```python
from build123d import *

# Parameters (mm, degrees)
CYLINDER042_R     = 3.15
CYLINDER042_DEPTH = 10
ARRAY016_Y_COUNT  = 2
ARRAY016_Y_PITCH  = 51.7
CYLINDER036_R     = 2.2
CYLINDER036_DEPTH = 26
ARRAY010_X_COUNT  = 2
ARRAY010_X_PITCH  = 11.9
ARRAY010_Y_COUNT  = 3
ARRAY010_Y_PITCH  = 7.5
CYLINDER035_R     = 2.2
CYLINDER035_DEPTH = 26
ARRAY009_X_COUNT  = 2
ARRAY009_X_PITCH  = 11.9
ARRAY009_Y_COUNT  = 3
ARRAY009_Y_PITCH  = 7.5
BOX041_W          = 26.3
BOX041_H          = 84
BOX041_DEPTH      = 8
BOX040_W          = 26.3
BOX040_H          = 144.8
BOX040_DEPTH      = 3.7


with BuildPart() as obj1:
    # Cylinder042 → Cylinder042 (new body)
    with BuildSketch(Plane(origin=(-15.15, -63.15, -71), x_dir=(1, 0, 0), z_dir=(0, 0, 1))):
        Circle(CYLINDER042_R)
    extrude(amount=CYLINDER042_DEPTH)

    # Array016 Y: obj1 ×2


with BuildPart() as obj1_1:
    add(obj1.part)
    with Locations(*[(0, -i * ARRAY016_Y_PITCH, 0) for i in range(1, ARRAY016_Y_COUNT)]):
        add(obj1.part)


with BuildPart() as taladros_cadera_centro1:
    # Cylinder036 → Cylinder036 (new body)
    with BuildSketch(Plane(origin=(-9.2, -39.8, -80), x_dir=(1, 0, 0), z_dir=(0, 0, 1))):
        Circle(CYLINDER036_R)
    extrude(amount=CYLINDER036_DEPTH)

    # Array010 X: Taladros_cadera_centro1 ×2


with BuildPart() as taladros_cadera_centro1_1:
    add(taladros_cadera_centro1.part)
    with Locations(*[(-i * ARRAY010_X_PITCH, 0, 0) for i in range(1, ARRAY010_X_COUNT)]):
        add(taladros_cadera_centro1.part)

    # Array010 Y: Taladros_cadera_centro1 ×3


with BuildPart() as taladros_cadera_centro1_2:
    add(taladros_cadera_centro1_1.part)
    with Locations(*[(0, i * ARRAY010_Y_PITCH, 0) for i in range(1, ARRAY010_Y_COUNT)]):
        add(taladros_cadera_centro1_1.part)


with BuildPart() as taladros_cadera_centro1_3:
    # Array010 placement: moved
    add(taladros_cadera_centro1_2.part.moved(Location((0, -113.4, 0))))


with BuildPart() as taladros_cadera_centro:
    # Cylinder035 → Cylinder035 (new body)
    with BuildSketch(Plane(origin=(-9.2, -39.8, -80), x_dir=(1, 0, 0), z_dir=(0, 0, 1))):
        Circle(CYLINDER035_R)
    extrude(amount=CYLINDER035_DEPTH)

    # Array009 X: Taladros_cadera_centro ×2


with BuildPart() as taladros_cadera_centro_1:
    add(taladros_cadera_centro.part)
    with Locations(*[(-i * ARRAY009_X_PITCH, 0, 0) for i in range(1, ARRAY009_X_COUNT)]):
        add(taladros_cadera_centro.part)

    # Array009 Y: Taladros_cadera_centro ×3


with BuildPart() as taladros_cadera_centro_2:
    add(taladros_cadera_centro_1.part)
    with Locations(*[(0, i * ARRAY009_Y_PITCH, 0) for i in range(1, ARRAY009_Y_COUNT)]):
        add(taladros_cadera_centro_1.part)


with BuildPart() as cadera_base_centro001:
    # Box041 → Box041 (new body)
    with BuildSketch(Plane(origin=(-28.3, -133, -70), x_dir=(1, 0, 0), z_dir=(0, 0, 1))):
        with Locations((13.15, 42)):
            Rectangle(BOX041_W, BOX041_H)
    extrude(amount=BOX041_DEPTH)


with BuildPart() as cadera_centro_full:
    # Box040 → Box040 (new body)
    with BuildSketch(Plane(origin=(-28.3, -163.4, -68), x_dir=(1, 0, 0), z_dir=(0, 0, 1))):
        with Locations((13.15, 72.4)):
            Rectangle(BOX040_W, BOX040_H)
    extrude(amount=BOX040_DEPTH)

    # Fusion009003047: union Cadera_base_centro001
    add(cadera_base_centro001.part)


with BuildPart() as cadera_centro_full_1:
    # Fusion009003047 placement: moved
    add(cadera_centro_full.part.moved(Location((0, 2, 0))))

    # Cut035: cut Taladros_cadera_centro
    add(taladros_cadera_centro_2.part, mode=Mode.SUBTRACT)

    # Cut036: cut Taladros_cadera_centro1
    add(taladros_cadera_centro1_3.part, mode=Mode.SUBTRACT)

    # Cut049: cut obj1
    add(obj1_1.part, mode=Mode.SUBTRACT)


solid = cadera_centro_full_1.part
```
Geometry check sheet. Reference: the model listing, model coordinates, mm. A direction names the side the tool comes from. Round coordinates to 2 decimals unless told otherwise and drop trailing zeros. Order: outer loops, then holes, each group sorted by start corner. A loop starts at its lowest first (then second) coordinate and runs counter-clockwise, first axis right, second up. Notation, with made-up numbers: M 37,14 L 52,14 A11 ccw 52,20 Z; hole C -15,-17 d6. An arc over 180 degrees is marked long. Answer as CSV lines item,"result".
1) Sectioned sample at D-D on y = -32.3. Record the cut outline in (x, z).
Entries:
outline,"M -28.3,-68 L -23.3,-68 L -23.3,-64.3 L -28.3,-64.3 Z; M -18.9,-68 L -11.4,-68 L -11.4,-64.3 L -18.9,-64.3 Z; M -7,-68 L -2,-68 L -2,-64.3 L -7,-64.3 Z"
2) Sectioned sample at B-B on z = -66. Give the number of separate pieces and of enclosed holes in the cut face, and give its area (3 significant figures).
Entries:
separate pieces,"1"
enclosed holes,"14"
area,"3,560 mm2"
3) Sectioned sample at C-C on x = -25.25. Record the cut outline in (y, z), and give its area (3 significant figures).
Entries:
outline,"M -161.4,-68 L -131,-68 L -131,-70 L -47,-70 L -47,-68 L -16.6,-68 L -16.6,-64.3 L -47,-64.3 L -47,-62 L -131,-62 L -131,-64.3 L -161.4,-64.3 Z"
area,"897 mm2"
4) Tool access check on faces 1 (the face through (-15, -146, -64.3)), 2 (the face through (-8.017, -30.445, -66.176)), 3 (the face through (-15, -32, -68)). Record the directions out of +Z, -Z, +X, -X, +Y, -Y that give a thin tool (end or side, any length) a straight path to the whole face; none if there is none.
Entries:
face 1,"+Z, +X, -X, -Y"
face 2,"+Z, -Z"
face 3,"-Z, +X, -X, +Y"
5) Thickness scan on probe 1 along Y at (x, z) = (-15.15, -63.75); probe 2 along X at (y, z) = (-145.7, -67.1); probe 3 along Y at (x, z) = (-12.5, -63). Record the ranges inside material, lowest first. Write a range as [from, to].
Entries:
probe 1,"[-131, -118], [-111.7, -66.3], [-60, -47]"
probe 2,"[-28.3, -23.3], [-18.9, -11.4], [-7, -2]"
probe 3,"[-131, -116.55], [-113.15, -64.85], [-61.45, -47]"
6) Gauge pin test, flat ends, axial feed: pin 1 Ø7 at (x, y) = (-21.1, -145.7) entering from -Z; pin 2 Ø13 at (x, y) = (-11.5, -142) entering from +Z; pin 3 Ø1 at (x, z) = (-24.5, -63.5) entering from -Y; pin 4 Ø3.5 at (x, y) = (-9.2, -39.8) entering from +Z. Record the tip position at first contact, or that the pin passes through.
Entries:
pin 1,"z = -68"
pin 2,"z = -64.3"
pin 3,"y = -131"
pin 4,"through"
7) Sectioned sample at A-A on y = -63.15. Record the cut outline in (x, z), and give its area (3 significant figures).
Entries:
outline,"M -28.3,-70 L -18.3,-70 L -18.3,-62 L -28.3,-62 Z; M -12,-70 L -2,-70 L -2,-62 L -12,-62 Z"
area,"160 mm2"
8) Mould release check, pull along Y, two halves, no side actions. Record for faces 4 (the face through (-15, -131, -63)), 5 (the face through (-8.017, -37.945, -66.176)), 6 (the face through (-7.168, -25.643, -66.176)), 7 (the face through (-15, -47, -63)): +Y half, -Y half, draft (parallel to the pull), parting line (faces both ways), or undercut.
Entries:
face 4,"-Y half"
face 5,"undercut"
face 6,"undercut"
face 7,"+Y half"
